Autodesk Inventor part; units mm, degrees
ref_plane "YZ Plane" through (0, 0, 0) normal (1, 0, 0) x (0, 1, 0)
ref_plane "XZ Plane" through (0, 0, 0) normal (0, 1, 0) x (-1, 0, 0)
ref_plane "XY Plane" through (0, 0, 0) normal (0, 0, 1) x (1, 0, 0)
sketch "Sketch1" plane through (0, 0, 0) normal (1, 0, 0) x (0, 1, 0)
  line L0 (0, 0) -> (-76.2, 0)
  line L1 (-76.2, 0) -> (-76.2, -685.8)
  line L2 (-76.2, -685.8) -> (0, -685.8)
  line L3 (0, -685.8) -> (0, 0)
  dimension "d0" = 76.2
  dimension "d1" = 685.8
extrude "Plate1" add sketch "Sketch1" along normal blind 3.175
sketch "Sketch2" plane through (0, -76.2, -3.175) normal (0, 0, 1) x (1, 0, 0)
  line L0 (0, 76.2) -> (0, 0)
  line L1 (0, 0) -> (127, 0)
  line L2 (127, 0) -> (127, 76.2)
  line L3 (127, 76.2) -> (0, 76.2)
edge flange "Flange1" height 127 angle 90 thickness 3.175 bend radius 3.175 thickness toward (0, 0, 1) relief tear relief width 3.175 relief depth 1.5875 edges at (3.175, -38.1, 0) wall of the first edge with corners at (0, 0, -3.175) (0, -76.2, -3.175) (127, -76.2, -3.175) (127, 0, -3.175)
bend "Bend1"
corner "Corner1"
sketch "Sketch3" plane through (3.175, 0, 0) normal (1, 0, 0) x (0, 0, -1)
  point P0 (0, 0)
equation "\"d3\" = BendReliefWidth"
equation "\"d4\" = BendReliefDepth"
equation "\"d5\" = MinimumRemnant"
equation "\"d6\" = BendRadius"
equation "\"d9\" = BendRadius"
equation "\"d10\" = CornerReliefSize"
equation "\"d11\" = GapSize"
equation "\"d12\" = JacobiRadiusSize"
equation "\"BendRadius\" = Thickness"
equation "\"BendReliefWidth\" = Thickness"
equation "\"BendReliefDepth\" = 0.5 * Thickness"
equation "\"CornerReliefSize\" = 4 * Thickness"
equation "\"MinimumRemnant\" = 2 * Thickness"
equation "\"TransitionRadius\" = BendRadius"
equation "\"JacobiRadiusSize\" = BendRadius"
equation "\"GapSize\" = Thickness"
equation "\"d2\" = BendRadius"
properties part number "ForkLift mockup"
Here's how the part is built. I have some questions about the finished solid (model axes, mm). A direction names the side the tool comes from. Round coordinates to 2 decimals unless told otherwise and drop trailing zeros. Order: outer loops, then holes, each group sorted by start corner. A loop starts at its lowest first (then second) coordinate and runs counter-clockwise, first axis right, second up. Notation, with made-up numbers: (-18.75, -40) -> (24.25, -40) arc R12 ccw to (24.25, -17) -> close; hole circle Ø9 at (24.25, 60.5). An arc over 180 degrees is marked (long way). Use a Markdown table: item, result. Add a question column.
(1) Suppose I cut it at B-B, the plane x = 24. Please give me the cut outline in (y, z) (3 decimals), and give its area (3 significant figures).
(2) I need wall thicknesses on line 1 along X through (y, z) = (-7, -551) (3 decimals); line 2 along Z through (x, y) = (62.5, -56) (3 decimals). Which ranges of each line are inside material? Lowest first, please.
(3) Suppose I cut it at C-C, the plane z = -357.5. Please give me the cut outline in (x, y) (3 decimals), and give its area (3 significant figures).
(4) For faces 1 (the face through (3.175, -39, -341)), 2 (the face through (3, 0, -341)), which set-ups out of +Z, -Z, +X, -X, +Y, -Y let a thin tool reach every point of the face, with its end or its side?
(5) For pin 1 Ø1.5 at (x, y) = (31, -44.5) entering from -Z (3 decimals), with a flat end and sliding along its axis, tell me the tip position at first contact or that it passes through.
(6) Suppose I cut it at A-A, the plane y = -43. Please give me the cut outline in (x, z) (3 decimals).
Verdict:
| question | item | result |
|---|---|---|
| 1 | outline | (-76.2, -3.175) -> (0, -3.175) -> (0, 0) -> (-76.2, 0) -> close |
| 1 | area | 242 mm2 |
| 2 | line 1 | 0 to 3.175 |
| 2 | line 2 | -3.175 to 0 |
| 3 | outline | (0, -76.2) -> (3.175, -76.2) -> (3.175, 0) -> (0, 0) -> close |
| 3 | area | 242 mm2 |
| 4 | face 1 | -Z, +X, +Y, -Y |
| 4 | face 2 | +Z, -Z, +X, -X, +Y |
| 5 | pin 1 | z = -3.175 |
| 6 | outline | (0, -685.8) -> (3.175, -685.8) -> (3.175, -6.35) arc R3.175 cw to (6.35, -3.175) -> (127, -3.175) -> (127, 0) -> (6.35, 0) arc R6.35 ccw to (0, -6.35) -> close |
